```python
from build123d import *

# Parameters (mm, degrees)
CUT_EXTRUDE1_DEPTH      = 271.724562794
CUT_EXTRUDE1_DEPTH_BACK = 271.724562794
SKETCH2_W               = 101.6
SKETCH2_H               = 25.4
SKETCH2_W_2             = 76.2


with BuildPart() as part:
    # Sketch1 → Revolve1 (revolve)
    with BuildSketch(Plane.XY):
        with BuildLine():
            Line((-207.01, 0), (207.01, 0))
            Line((207.01, 0), (257.81, 0))
            ThreePointArc((257.81, 0), (243.872346186, 34.954362155), (209.707345133, 50.728338522))
            Line((209.707345133, 50.728338522), (66.601946903, 58.337589301))
            ThreePointArc((66.601946903, 58.337589301), (62.855469091, 58.416444431), (59.111643192, 58.254945923))
            Line((59.111643192, 58.254945923), (-209.871971831, 37.992356037))
            ThreePointArc((-209.871971831, 37.992356037), (-234.944307999, 25.909157389), (-245.11, 0))
            Line((-245.11, 0), (-207.01, 0))
        make_face()
    revolve(axis=Axis((-207.01, 0, 0), (1, 0, 0)))

    # Sketch2 → Cut-Extrude1 (cut, two sides: drawn at the far end of the back side and taken through both)
    with BuildSketch(Plane(origin=(0, 0, 0), x_dir=(1, 0, 0), z_dir=(0, 1, 0)).offset(-CUT_EXTRUDE1_DEPTH_BACK)):
        with Locations((207.01, 0)):
            Rectangle(SKETCH2_W, SKETCH2_H)
        with Locations((-207.01, 0)):
            Rectangle(SKETCH2_W_2, SKETCH2_H)
    extrude(amount=CUT_EXTRUDE1_DEPTH + CUT_EXTRUDE1_DEPTH_BACK, mode=Mode.SUBTRACT)


solid = part.part
```
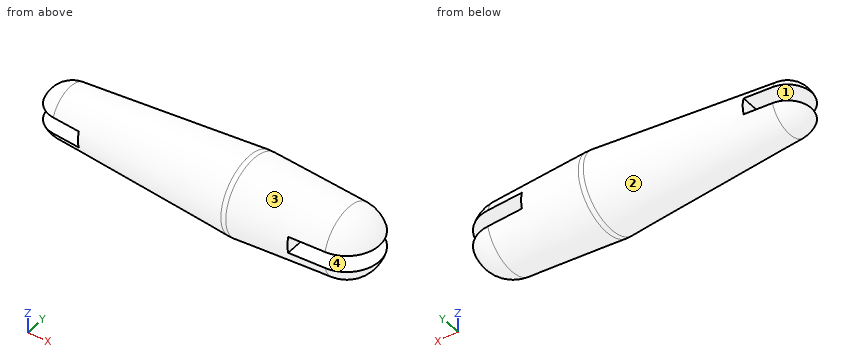
Geometry: final body of the model. Coordinates: model frame, mm. Face numbers are marked on the shaded views. A direction names the side the tool comes from. Give positions to 0.01 mm unless a question says otherwise; leave off trailing zeros. Loops run counter-clockwise (first coordinate to the right, second up) from the corner with the lowest first, then second, coordinate; pieces in that order, holes last. Notation, with made-up numbers: (68.5, 13.5) -> (108.5, 13.5) arc R22 cw to (108.5, 47.5) -> close; hole circle Ø9 at (24.5, -36). An arc over 180 degrees is marked (long way). Use one line per item in the form item = value.
Item 1: Access query for the marked faces 3 and 4. Directions: +Z, -Z, +X, -X, +Y, -Y. A direction counts if a zero-diameter tool reaches every point of the face in a straight line with its end or side. Return the directions, or none.
A:
face_3 = +X
face_4 = +X, +Y, -Y
Item 2: Section query B-B on x = -119. Output: boundary loops of the cut face in (y, z).
A:
outline = circle Ø89.68 at (0, 0)
Item 3: Pin query (flat end, axial travel): P1, Ø8, axis at x = -175.5, y = 32.5, coming from the +Z side; P2, Ø12, axis at x = -138, z = 15.5, coming from the +Y side; P3, Ø12.5, axis at y = 10.5, z = -0.5, coming from the -X side. Return the tip coordinate at first contact, or that it passes through.
A:
P1 = 28.91
P2 = 42.43
P3 = -168.91
Item 4: Draft query along Z for the marked faces 1 and 2. Return one class per face: pulls with the +Z half, pulls with the -Z half, needs draft (parallel to the pull), parting line crosses it, or undercut.
A:
face_1 = undercut
face_2 = parting line crosses it
Item 5: Line query: probe 1 along Z at (x, y) = (-183.5, -21.5); probe 2 along Z at (x, y) = (-26.5, 7.5); probe 3 along Z at (x, y) = (-175, 22.5). Output: solid intervals per line, ascending.
A:
probe_1 = -33.71 to -12.7, 12.7 to 33.71
probe_2 = -51.26 to 51.26
probe_3 = -33.82 to -12.7, 12.7 to 33.82
Item 6: Section query A-A on x = 219. Output: boundary loops of the cut face in (y, z), and give its area (3 significant figures).
A:
outline = (-47.7, -12.7) arc R49.36 ccw to (47.7, -12.7) -> close; (-47.7, 12.7) -> (47.7, 12.7) arc R49.36 ccw to start
area = 5,180 mm^2
